Work out the finished part from the listing and answer in its coordinate system (mm). A direction names the side the tool comes from. Coordinates: 2 decimals unless noted, no trailing zeros. Write each loop counter-clockwise with the first axis right and the second up, starting at its lowest first coordinate (ties: lowest second). Pieces come first, ordered by that corner, then holes. Notation, with made-up numbers: (21.25, 77) - (75.25, 77) arc R3 ccw to (75.25, 82) - close; hole circle Ø10 at (-2.5, -35.5). An arc over 180 degrees is marked (long way). Use one line per item in the form item = value. Start each with the question number.
Item 1: Consider probe 1 along Y at (x, z) = (7.25, -2.5); probe 2 along Y at (x, z) = (-2, 4.5); probe 3 along X at (y, z) = (11, 2.25). Determine where each line is inside the solid, lowest interval first.
Item 2: For faces 1 (the cylindrical face through (3.905, 3.542, 0.867)), 2 (the flat face through (0, 17.5, 0)), determine the directions among +Z, -Z, +X, -X, +Y, -Y from which every point of the face is accessible in a straight line to the end or side of a thin tool.
Item 3: Given pin 1 (4 mm diameter, centred on y = 13.5, z = 2, fed in from -X); pin 2 (1.5 mm diameter, centred on y = 13.5, z = 7, fed in from -X); pin 3 (6 mm diameter, centred on y = 9.5, z = 5.5, fed in from -X); pin 4 (8 mm diameter, centred on y = 4.5, z = 6, fed in from +X), each flat-ended and moving along its own axis, determine where each tip first touches the part or whether it passes through.
Item 4: A cutting plane is placed at A-A (x = 0). Write down the section's boundary in (y, z).
Item 5: A cutting plane is placed at B-B (z = 0). Write down the section's boundary in (x, y).
Item 6: A cutting plane is placed at C-C (y = 7.5). Write down the section's boundary in (x, z).
from build123d import *


with BuildPart() as part:
    # Esquisse1 → Base-Révolution (revolve)
    with BuildSketch(Plane.XY, mode=Mode.PRIVATE) as base_r_volution_sk:
        with BuildLine():
            Line((0, 0), (3.5, 0))
            Line((3.5, 0), (4, 0.5))
            Line((4, 0.5), (4, 6.5))
            ThreePointArc((4, 6.5), (4.3, 6.8), (4.6, 6.5))
            Line((4.6, 6.5), (6, 6.5))
            Line((6, 6.5), (6, 14.5))
            ThreePointArc((6, 14.5), (6.3, 14.8), (6.6, 14.5))
            Line((6.6, 14.5), (10, 14.5))
            Line((10, 14.5), (10, 16.5))
            Line((10, 16.5), (9, 17.5))
            Line((9, 17.5), (0, 17.5))
            Line((0, 17.5), (0, 0))
        make_face()
    revolve(base_r_volution_sk.sketch.rotate(Axis((0, 0, 0), (0, 1, 0)), 90), axis=Axis((0, 0, 0), (0, 1, 0)))


solid = part.part
Answer:
q1.probe_1 = 14.5 to 17.5
q1.probe_2 = 6.5 to 17.5
q1.probe_3 = -5.56 to 5.56
q2.face_1 = -Y
q2.face_2 = +Z, -Z, +X, -X, +Y
q3.pin_1 = -10
q3.pin_2 = through
q3.pin_3 = -5.45
q3.pin_4 = 5.44
q4.outline = (0, -3.5) - (0.5, -4) - (6.5, -4) arc R0.3 cw to (6.5, -4.6) - (6.5, -6) - (14.5, -6) arc R0.3 cw to (14.5, -6.6) - (14.5, -10) - (16.5, -10) - (17.5, -9) - (17.5, 9) - (16.5, 10) - (14.5, 10) - (14.5, 6.6) arc R0.3 cw to (14.5, 6) - (6.5, 6) - (6.5, 4.6) arc R0.3 cw to (6.5, 4) - (0.5, 4) - (0, 3.5) - close
q5.outline = (-10, 14.5) - (-6.6, 14.5) arc R0.3 cw to (-6, 14.5) - (-6, 6.5) - (-4.6, 6.5) arc R0.3 cw to (-4, 6.5) - (-4, 0.5) - (-3.5, 0) - (3.5, 0) - (4, 0.5) - (4, 6.5) arc R0.3 cw to (4.6, 6.5) - (6, 6.5) - (6, 14.5) arc R0.3 cw to (6.6, 14.5) - (10, 14.5) - (10, 16.5) - (9, 17.5) - (-9, 17.5) - (-10, 16.5) - close
q6.outline = circle Ø12 at (0, 0)
